Here's how the part is built. I have some questions about the finished solid (model axes, mm). Round coordinates to 2 decimals unless told otherwise and drop trailing zeros. Order: outer loops, then holes, each group sorted by start corner. A loop starts at its lowest first (then second) coordinate and runs counter-clockwise, first axis right, second up.
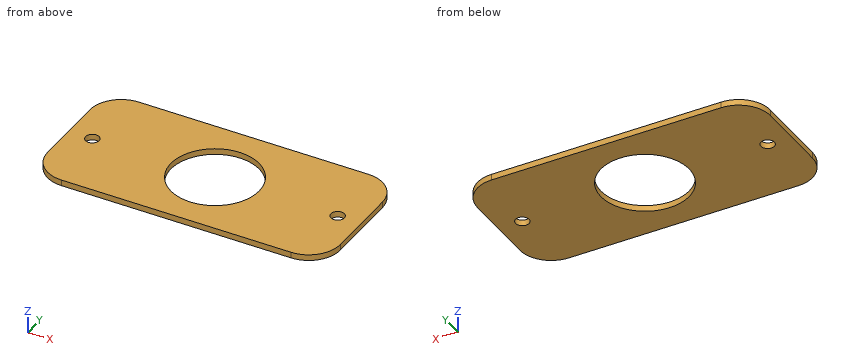
```python
from build123d import *

# Parameters (mm, degrees)
ESQUISSE1_W          = 74
ESQUISSE1_H          = 35
ESQUISSE1_R          = 11.15
ESQUISSE1_R_2        = 1.5
BOSS_EXTRU_1_DEPTH   = 1.5
D_GAGEMENT_M31_D     = 3.4
D_GAGEMENT_M31_DEPTH = 1.5
CONG_1_R             = 8


with BuildPart() as part:
    # Esquisse1 → Boss.-Extru.1 (new body)
    with BuildSketch(Plane.XY):
        with Locations((37, 17.5)):
            Rectangle(ESQUISSE1_W, ESQUISSE1_H)
        with Locations((37, 17.5)):
            Circle(ESQUISSE1_R, mode=Mode.SUBTRACT)
        with Locations((6, 17.5)):
            Circle(ESQUISSE1_R_2, mode=Mode.SUBTRACT)
        with Locations((68, 17.5)):
            Circle(ESQUISSE1_R_2, mode=Mode.SUBTRACT)
    extrude(amount=BOSS_EXTRU_1_DEPTH)

    # Dégagement M31
    with Locations(Plane.XY.offset(1.5)):
        with Locations((6, 17.5), (68, 17.5)):
            Hole(D_GAGEMENT_M31_D / 2, depth=D_GAGEMENT_M31_DEPTH)

    # Congé1
    cong_1_edges = [part.edges().sort_by_distance(p)[0] for p in [
        (0, 35, 0.75),
        (74, 35, 0.75),
        (74, 0, 0.75),
        (0, 0, 0.75),
    ]]
    fillet(cong_1_edges, radius=CONG_1_R)


solid = part.part
```
1. If we section it at D-D, the plane y = 22: Write out the boundary of the cut face in (x, z).
Evaluation:
outline: (0, 0) - (26.8, 0) - (26.8, 1.5) - (0, 1.5) - close; (47.2, 0) - (74, 0) - (74, 1.5) - (47.2, 1.5) - close
2. I need wall thicknesses on probe 1 along Y at (x, z) = (6, 1.1); probe 2 along X at (y, z) = (7.5, 1.15); probe 3 along X at (y, z) = (23, 0.4). Which ranges of each line are inside material? Lowest first, please.
Evaluation:
probe 1: y = 0.25 to 15.8, 19.2 to 34.75
probe 2: x = 0.02 to 32.07, 41.93 to 73.98
probe 3: x = 0 to 27.3, 46.7 to 74
3. If we section it at C-C, the plane x = 37: Write out the boundary of the cut face in (y, z), and give its area (4 significant figures).
Evaluation:
outline: (0, 0) - (6.35, 0) - (6.35, 1.5) - (0, 1.5) - close; (28.65, 0) - (35, 0) - (35, 1.5) - (28.65, 1.5) - close
area: 19.05 mm2
4. If we section it at A-A, the plane y = 17.5: Write out the boundary of the cut face in (x, z), and give its area (4 significant figures).
Evaluation:
outline: (0, 0) - (4.3, 0) - (4.3, 1.5) - (0, 1.5) - close; (7.7, 0) - (25.85, 0) - (25.85, 1.5) - (7.7, 1.5) - close; (48.15, 0) - (66.3, 0) - (66.3, 1.5) - (48.15, 1.5) - close; (69.7, 0) - (74, 0) - (74, 1.5) - (69.7, 1.5) - close
area: 67.35 mm2
5. If we section it at B-B, the plane z = 0.85: Write out the boundary of the cut face in (x, y).
Evaluation:
outline: (0, 8) arc R8 ccw to (8, 0) - (66, 0) arc R8 ccw to (74, 8) - (74, 27) arc R8 ccw to (66, 35) - (8, 35) arc R8 ccw to (0, 27) - close; hole circle Ø3.4 at (6, 17.5); hole circle Ø22.3 at (37, 17.5); hole circle Ø3.4 at (68, 17.5)
